For this review, take the finished solid that the model builds, in its own axes (mm). Face numbers are marked on the shaded views. A direction names the side the tool comes from. Give positions to 0.01 mm unless a question says otherwise; leave off trailing zeros. Order: outer loops, then holes, each group sorted by start corner. A loop starts at its lowest first (then second) coordinate and runs counter-clockwise, first axis right, second up. Notation, with made-up numbers: (42.5, 19) -> (49.5, 19) arc R16 ccw to (49.5, 47) -> close; hole circle Ø5 at (-10, 48.5). An arc over 180 degrees is marked (long way). One line per item, written item: value. Start each with the question number.
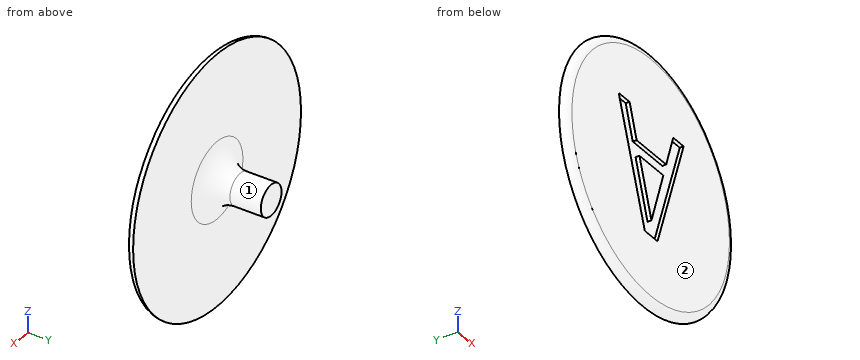
Autodesk Inventor part; units mm, degrees
ref_plane "YZ Plane" through (0, 0, 0) normal (1, 0, 0) x (0, 1, 0)
ref_plane "XZ Plane" through (0, 0, 0) normal (0, 1, 0) x (-1, 0, 0)
ref_plane "XY Plane" through (0, 0, 0) normal (0, 0, 1) x (1, 0, 0)
sketch "Sketch1" plane through (0, 0, 0) normal (0, 1, 0) x (-1, 0, 0)
  circle A0 centre (0, 0) radius 32.5
  dimension "d0" = 65
extrude "Extrusion3" add sketch "Sketch1" along normal blind 2
sketch "Sketch3" plane through (0, 2, 0) normal (0, 1, 0) x (1, 0, 0)
  circle A0 centre (0, 0) radius 4
  dimension "d17" = 8
extrude "Extrusion4" add sketch "Sketch3" along normal blind 14
fillet "Fillet2" radius 6 1 edges at (-4, 2, 0)
fillet "Fillet3" radius 2 1 edges at (32.5, 0, 0)
sketch "Sketch4" plane through (0, 0, 0) normal (0, -1, 0) x (1, 0, 0)
  line L0 (32.5, -32.5) -> (-32.5, -32.5) construction
  line L1 (-32.5, -32.5) -> (-32.5, 32.5) construction
  line L2 (-32.5, 32.5) -> (32.5, 32.5) construction
  line L3 (32.5, 32.5) -> (32.5, -32.5) construction
  line L4 (32.5, 32.5) -> (-32.5, 32.5)
  line L5 (-32.5, 32.5) -> (-32.5, -32.5)
  line L6 (-32.5, -32.5) -> (32.5, -32.5)
  line L7 (32.5, -32.5) -> (32.5, 32.5)
  circle A0 centre (0, 0) radius 4
  line L8 (32.5, 32.5) -> (-32.5, -32.5) construction
  line L9 (-32.5, 32.5) -> (32.5, -32.5) construction
  line L10 (12.7634, 15) -> (2.6499, -15)
  line L11 (2.6499, -15) -> (-2.2609, -15)
  line L12 (-2.2609, -15) -> (-12.3744, 15)
  line L13 (-12.3744, 15) -> (-8.1686, 15)
  line L14 (-8.1686, 15) -> (-5.4457, 6.6126)
  line L15 (-5.4457, 6.6126) -> (6.0049, 6.6126)
  line L16 (6.0049, 6.6126) -> (8.7277, 15)
  line L17 (8.7277, 15) -> (12.7634, 15)
  line L18 (-4.3517, 3.2091) -> (0.2917, -10.9157)
  line L19 (0.2917, -10.9157) -> (4.9109, 3.2091)
  line L20 (4.9109, 3.2091) -> (-4.3517, 3.2091)
  dimension "d22" = 65
  dimension "d23" = 65
  dimension "d24" = 65
  dimension "d25" = 65
  dimension "d26" = 0
  dimension "d27" = 0
emboss "Emboss2" sketch "Sketch4" operation cut depth 1 direction (0, 1, 0) contours A0 L19 | L20 A0 | A0 L18 | L10 L11 L12 L13 L14 L15 L16 L17
properties part number "Stepper_Closing_1"
Q1. For the marked faces 1 and 2, list the 3-axis set-ups (+Z, -Z, +X, -X, +Y, -Y) from which the entire face can be reached by the end or side of a thin tool; tool diameter is ignored.
Q2. For pin 1 Ø0.8 at (x, y) = (-11, 0.5) entering from -Z; pin 2 Ø1.1 at (x, y) = (-0.5, 0.5) entering from -Z; pin 3 Ø10 at (x, z) = (-17, 24.5) entering from -Y; pin 4 Ø0.5 at (x, y) = (10, 0.5) entering from -Z, all flat-tipped, find the tip position at first contact; note any pin that passes through.
Q3. For line 1 along Y through (x, z) = (22, 13); line 2 along X through (y, z) = (12.5, 0); line 3 along Y through (x, z) = (-17.5, -26), list the stretches that pass through material, from the lowest coordinate up.
Q4. Take a section at C-C (y = 3.5). State the section outline as (x, z) points, and give its area (3 significant figures).
Q5. Take a section at A-A (y = 9). State the section outline as (x, z) points, and give its area (3 significant figures).
Answers below:
1. face 1: +Y
1. face 2: +Z, -Z, +X, -X, -Y
2. pin 1: stops at z = -30.27
2. pin 2: stops at z = -32.26
2. pin 3: stops at y = 0
2. pin 4: stops at z = -30.48
3. line 1: y = 0 to 2
3. line 2: x = -4 to 4
3. line 3: y = 0.19 to 2
4. outline: circle Ø12.06 at (0, 0)
4. area: 114 mm²
5. outline: circle Ø8 at (0, 0)
5. area: 50.3 mm²
